The model under review builds one solid part; all positions refer to its coordinate system, in mm. Face numbers are marked on the shaded views. A direction names the side the tool comes from. Round coordinates to 2 decimals unless told otherwise and drop trailing zeros. Write each loop counter-clockwise with the first axis right and the second up, starting at its lowest first coordinate (ties: lowest second). Pieces come first, ordered by that corner, then holes. Notation, with made-up numbers: M 16.5,73 L 56.5,73 A30 cw 56.5,105 Z; hole C -12,-21.5 d8. An arc over 180 degrees is marked long. One line per item, written item: value. Start each with the question number.
1) Wall thickness on probe 1 along Y at (x, z) = (0, 0.85); probe 2 along Y at (x, z) = (0, -1); probe 3 along Y at (x, z) = (0, -0.45): over which ranges is each line inside the solid? List them lowest first.
2) Tool access review of the marked faces 1 and 2: name each direction out of +Z, -Z, +X, -X, +Y, -Y from which nothing blocks a thin tool from reaching the whole face with its end or side.
3) Take a section at D-D, the plane y = 7. Write out the cut boundary in (x, z).
4) Take a section at A-A, the plane x = 0. Write out the cut boundary in (y, z).
5) Take a section at C-C, the plane z = -0.25. Write out the cut boundary in (x, y), and give its area (3 significant figures).
6) For P1, Ø1.6, axis at x = 0, y = 6, coming from the -Z side; P2, Ø0.6, axis at x = -0.5, y = 1.5, coming from the -Z side, all flat-tipped, find the tip position at first contact; note any pin that passes through.
7) Mouldability with a two-part tool opening along X and no side actions: class the marked faces 3, 4 and 5 as +X half, -X half, draft (parallel to the pull), parting line (faces both ways), or undercut.
8) Take a section at B-B, the plane y = 1.5. Write out the cut boundary in (x, z).
from build123d import *

# Parameters (mm, degrees)
SKETCH_1_W          = 8
SKETCH_1_H          = 3
EXTRUDE_1_DEPTH     = 3
SKETCH_2_W          = 8
SKETCH_2_H          = 8
EXTRUDE_2_DEPTH     = 3
SKETCH_2_3_R        = 2.6
CUT_EXTRUDE_1_DEPTH = 0.8
SKETCH_3_R          = 0.6
CUT_EXTRUDE_2_DEPTH = 13.083045974
SKETCH_3_3_R        = 1
CUT_EXTRUDE_3_DEPTH = 1.5


with BuildPart() as part:
    # 草图1 → 凸台-拉伸1 (new body)
    with BuildSketch(Plane(origin=(0, 0, 0), x_dir=(1, 0, 0), z_dir=(0, 1, 0))):
        Rectangle(SKETCH_1_W, SKETCH_1_H)
    extrude(amount=EXTRUDE_1_DEPTH)

    # 草图2 → 凸台-拉伸2 (add)
    with BuildSketch(Plane(origin=(0, 0, -1.5), x_dir=(-1, 0, 0), z_dir=(0, 0, -1))):
        with Locations((0, 7)):
            Rectangle(SKETCH_2_W, SKETCH_2_H)
    extrude(amount=-EXTRUDE_2_DEPTH)

    # 草图2<3> → 切除-拉伸1 (cut)
    with BuildSketch(Plane(origin=(0, 0, -1.5), x_dir=(-1, 0, 0), z_dir=(0, 0, -1))):
        with Locations((0, 7)):
            Circle(SKETCH_2_3_R)
    extrude(amount=-CUT_EXTRUDE_1_DEPTH, mode=Mode.SUBTRACT)

    # 草图3 → 切除-拉伸2 (cut, through all)
    with BuildSketch(Plane(origin=(0, 0, -1.5), x_dir=(-1, 0, 0), z_dir=(0, 0, -1))):
        with Locations((0, 1.5)):
            Circle(SKETCH_3_R)
    extrude(amount=-CUT_EXTRUDE_2_DEPTH, mode=Mode.SUBTRACT)

    # 草图3<3> → 切除-拉伸3 (cut)
    with BuildSketch(Plane(origin=(0, 0, -1.5), x_dir=(-1, 0, 0), z_dir=(0, 0, -1))):
        with Locations((0, 1.5)):
            Circle(SKETCH_3_3_R)
    extrude(amount=-CUT_EXTRUDE_3_DEPTH, mode=Mode.SUBTRACT)


solid = part.part
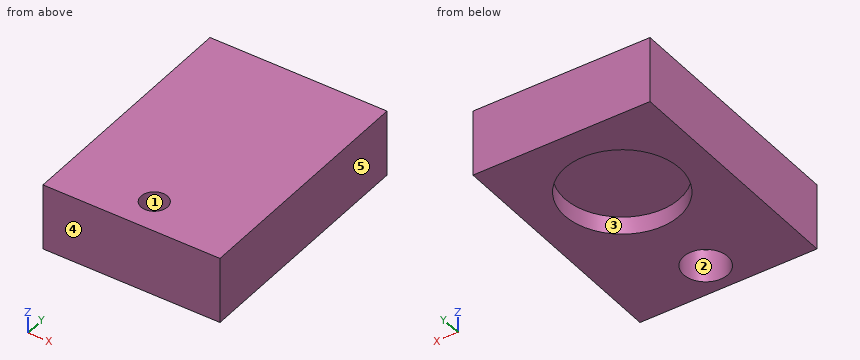
Checked values:
1. probe 1: y = 0 to 0.9, 2.1 to 11
1. probe 2: y = 0 to 0.5, 2.5 to 4.4, 9.6 to 11
1. probe 3: y = 0 to 0.5, 2.5 to 11
2. face 1: +Z, -Z
2. face 2: -Z
3. outline: M -4,-1.5 L -2.6,-1.5 L -2.6,-0.7 L 2.6,-0.7 L 2.6,-1.5 L 4,-1.5 L 4,1.5 L -4,1.5 Z
4. outline: M 0,-1.5 L 0.5,-1.5 L 0.5,0 L 0.9,0 L 0.9,1.5 L 0,1.5 Z; M 2.1,0 L 2.5,0 L 2.5,-1.5 L 4.4,-1.5 L 4.4,-0.7 L 9.6,-0.7 L 9.6,-1.5 L 11,-1.5 L 11,1.5 L 2.1,1.5 Z
5. outline: M -4,0 L 4,0 L 4,11 L -4,11 Z; hole C 0,1.5 d2
5. area: 84.9 mm2
6. P1: stops at z = -0.7
6. P2: stops at z = 0
7. face 3: undercut
7. face 4: draft
7. face 5: +X half
8. outline: M -4,-1.5 L -1,-1.5 L -1,0 L -0.6,0 L -0.6,1.5 L -4,1.5 Z; M 0.6,0 L 1,0 L 1,-1.5 L 4,-1.5 L 4,1.5 L 0.6,1.5 Z
